Part model, mm, in its own coordinate system. Face numbers are marked on the shaded views. A direction names the side the tool comes from. Round coordinates to 2 decimals unless told otherwise and drop trailing zeros. Write each loop counter-clockwise with the first axis right and the second up, starting at its lowest first coordinate (ties: lowest second). Pieces come first, ordered by that corner, then holes. Notation, with made-up numbers: (38.25, -21.5) -> (53.25, -21.5) arc R18 ccw to (53.25, -2.5) -> close; hole circle Ø8 at (-9.75, -33.75). An arc over 180 degrees is marked (long way). Return JSON: item names as keys, results as strings. Group by question number.
(1) Drop flat-ended pins along their axis: pin 1 Ø8 at (x, y) = (-3, -8.5) entering from -Z; pin 2 Ø3 at (y, z) = (1, 2.5) entering from +X; pin 3 Ø6 at (x, z) = (-12.5, -1.5) entering from +Y. Give the stop position or say it passes through.
(2) Saw through at A-A (x = 11.5). List the corners of the cut face in (y, z), plus the area to 3 significant figures.
(3) Saw through at B-B (y = 0). List the corners of the cut face in (x, z), plus the area to 3 significant figures.
(4) Tool access for the marked faces 5, 6, 7, 8 and 9: list every direction of +Z, -Z, +X, -X, +Y, -Y with a clear straight run to the whole face (end or side of a thin tool).
(5) Saw through at C-C (x = 16.5). List the corners of the cut face in (y, z), plus the area to 3 significant figures.
(6) Drill centre lines: L1, parallel to Y at x = 0, z = -1.75; L2, parallel to X at y = 17, z = 4; L3, parallel to Z at x = -15, y = 3. Where is each one in solid material? Low to high. Write a range as from..to.
(7) Mould opens along X. For the marked faces 1, 2, 3 and 4 say: +X half, -X half, draft (parallel to the pull), parting line (faces both ways), or undercut.
(8) Saw through at D-D (y = 16). List the corners of the cut face in (x, z).
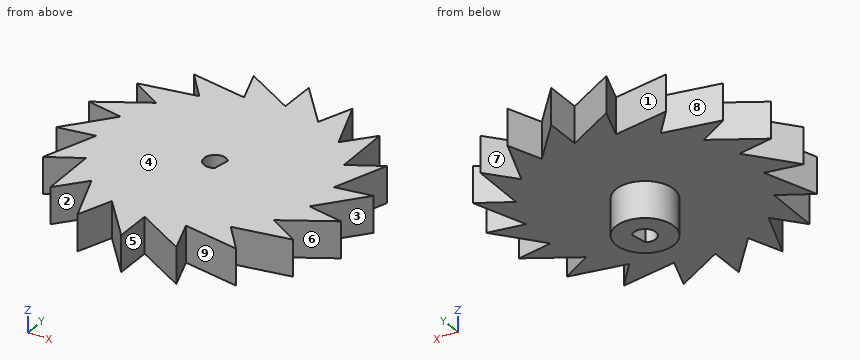
from build123d import *

# Parameters (mm, degrees)
BOSS_EXTRUDE1_DEPTH = 5
CIRPATTERN1_COUNT   = 18
SKETCH7_R           = 4
BOSS_EXTRUDE3_DEPTH = 5
CUT_EXTRUDE1_DEPTH  = 10


with BuildPart() as part:
    # Sketch1 → Boss-Extrude1 (new body)
    with BuildSketch(Plane.XY):
        Polygon((0, 0), (0, 20), (5.13030215, 14.095389312), align=None)
    boss_extrude1 = extrude(amount=BOSS_EXTRUDE1_DEPTH)

    # CirPattern1: Boss-Extrude1 ×18 about axis
    cirpattern1_axis = Axis((0, 0, 0), (0, 0, 1))
    for i in range(1, CIRPATTERN1_COUNT):
        add(boss_extrude1.rotate(cirpattern1_axis, i * 360 / CIRPATTERN1_COUNT))

    # Sketch7 → Boss-Extrude3 (add)
    with BuildSketch(Plane(origin=(0, 0, 0), x_dir=(-1, 0, 0), z_dir=(0, 0, -1))):
        Circle(SKETCH7_R)
    extrude(amount=BOSS_EXTRUDE3_DEPTH)

    # Sketch5 → Cut-Extrude1 (cut)
    with BuildSketch(Plane.XY.offset(5)):
        with BuildLine():
            Line((1.17901122, 0.927325479), (0.790582224, -1.274746935))
            ThreePointArc((0.790582224, -1.274746935), (-1.477195083, 0.260566092), (1.17901122, 0.927325479))
        make_face()
    extrude(amount=-CUT_EXTRUDE1_DEPTH, mode=Mode.SUBTRACT)


solid = part.part
Computed values:
{
 "1": {"pin 1": "z = 0", "pin 2": "x = 18.91", "pin 3": "y = 15.32"},
 "2": {"outline": "(-15.11, 0) -> (-13.71, 0) -> (-13.71, 5) -> (-15.11, 5) -> close; (-11.13, 0) -> (13.71, 0) -> (13.71, 5) -> (-11.13, 5) -> close", "area": "131 mm2"},
 "3": {"outline": "(-16.88, 0) -> (-4, 0) -> (-4, -5) -> (-1.5, -5) -> (-1.5, 5) -> (-16.88, 5) -> close; (1.02, -5) -> (4, -5) -> (4, 0) -> (16.88, 0) -> (16.88, 5) -> (1.02, 5) -> close", "area": "184 mm2"},
 "4": {"face 5": "+Z, -Z, -Y", "face 6": "+Z, -Z, +X", "face 7": "+Z, -Z, +Y", "face 8": "+Z, -Z, -X", "face 9": "+Z, -Z"},
 "5": {"outline": "(-10.16, 0) -> (-9.53, 0) -> (-9.53, 5) -> (-10.16, 5) -> close; (-5.39, 0) -> (-2.91, 0) -> (-2.91, 5) -> (-5.39, 5) -> close; (-0.47, 0) -> (2.91, 0) -> (2.91, 5) -> (-0.47, 5) -> close; (7.62, 0) -> (9.53, 0) -> (9.53, 5) -> (7.62, 5) -> close", "area": "42.0 mm2"},
 "6": {"L1": "-4..-1.5, 1.5..4", "L2": "-6.19..-3.61, 0..2.61, 6.19..7.53", "L3": "0..5"},
 "7": {"face 1": "undercut", "face 2": "undercut", "face 3": "+X half", "face 4": "draft"},
 "8": {"outline": "(-5.82, 0) -> (-1.8, 0) -> (-1.8, 5) -> (-5.82, 5) -> close; (0, 0) -> (3.48, 0) -> (3.48, 5) -> (0, 5) -> close; (5.82, 0) -> (7.91, 0) -> (7.91, 5) -> (5.82, 5) -> close"}
}
